from build123d import *

# Parameters (mm, degrees)
BOSS_EXTRUDE1_DEPTH = 10
CUT_EXTRUDE4_DEPTH  = 5
SKETCH7_R           = 4.5
CUT_EXTRUDE5_DEPTH  = 5
CUT_EXTRUDE6_DEPTH  = 10
CUT_EXTRUDE7_START  = -2
CUT_EXTRUDE7_DEPTH  = 2
SKETCH11_R          = 2.5
CUT_EXTRUDE8_DEPTH  = 104.25938214


with BuildPart() as part:
    # Sketch1 → Boss-Extrude1 (new body)
    with BuildSketch(Plane(origin=(0, 0, 0), x_dir=(1, 0, 0), z_dir=(0, 1, 0))):
        with BuildLine():
            Line((-32.5, 65), (-32.5, -65))
            ThreePointArc((-32.5, -65), (0, -97.5), (32.5, -65))
            Line((32.5, -65), (32.5, 65))
            ThreePointArc((32.5, 65), (0, 97.5), (-32.5, 65))
        make_face()
    extrude(amount=BOSS_EXTRUDE1_DEPTH)

    # Sketch6 → Cut-Extrude4 (cut)
    with BuildSketch(Plane(origin=(0, 10, 0), x_dir=(1, 0, 0), z_dir=(0, 1, 0))):
        with BuildLine():
            Line((-25, -65), (-25, 25))
            Line((-25, 25), (25, 25))
            Line((25, 25), (25, -65))
            ThreePointArc((25, -65), (0, -90), (-25, -65))
        make_face()
    extrude(amount=-CUT_EXTRUDE4_DEPTH, mode=Mode.SUBTRACT)

    # Sketch7 → Cut-Extrude5 (cut)
    with BuildSketch(Plane(origin=(0, 5, 0), x_dir=(1, 0, 0), z_dir=(0, 1, 0))):
        with Locations(Location((0, -65, 0), (0, 0, 270))):
            Circle(SKETCH7_R)
    extrude(amount=-CUT_EXTRUDE5_DEPTH, mode=Mode.SUBTRACT)

    # Sketch8 → Cut-Extrude6 (cut)
    with BuildSketch(Plane(origin=(0, 5, 0), x_dir=(1, 0, 0), z_dir=(0, 1, 0))):
        with BuildLine():
            Line((-16, -65), (-11, -65))
            ThreePointArc((-11, -65), (-7.778174593, -72.778174593), (0, -76))
            Line((0, -76), (0, -81))
            ThreePointArc((0, -81), (-11.313708499, -76.313708499), (-16, -65))
        make_face()
    extrude(amount=-CUT_EXTRUDE6_DEPTH, mode=Mode.SUBTRACT)

    # Sketch9 → Cut-Extrude7 (cut)
    with BuildSketch(Plane(origin=(0, 10, 0), x_dir=(1, 0, 0), z_dir=(0, 1, 0)).offset(CUT_EXTRUDE7_START)):
        with BuildLine():
            Line((-32.5, -65), (-30.5, -65))
            ThreePointArc((-30.5, -65), (0, -95.5), (30.5, -65))
            Line((30.5, -65), (32.5, -65))
            ThreePointArc((32.5, -65), (0, -97.5), (-32.5, -65))
        make_face()
        with BuildLine():
            Line((-30.5, 65), (-32.5, 65))
            ThreePointArc((-32.5, 65), (0, 97.5), (32.5, 65))
            Line((32.5, 65), (30.5, 65))
            ThreePointArc((30.5, 65), (0, 95.5), (-30.5, 65))
        make_face()
    extrude(amount=CUT_EXTRUDE7_DEPTH, mode=Mode.SUBTRACT)

    # Sketch11 → Cut-Extrude8 (cut, through all)
    with BuildSketch(Plane(origin=(0, 10, 0), x_dir=(1, 0, 0), z_dir=(0, 1, 0))):
        with Locations(Location((26, 32.5, 0), (0, 0, 270))):
            Circle(SKETCH11_R)
        with Locations(Location((-26, 32.5, 0), (0, 0, 270))):
            Circle(SKETCH11_R)
    extrude(amount=-CUT_EXTRUDE8_DEPTH, mode=Mode.SUBTRACT)


solid = part.part
Check sheet for the modelled part. Datum: model origin and axes. Units: mm. A direction names the side the tool comes from. Round coordinates to 2 decimals unless told otherwise and drop trailing zeros. Loops run counter-clockwise (first coordinate to the right, second up) from the corner with the lowest first, then second, coordinate; pieces in that order, holes last. Notation, with made-up numbers: M 79,22 L 101,22 A21 cw 101,50 Z; hole C 69.25,40.5 d4. An arc over 180 degrees is marked long. One line per question, with ' | ' between items. Start each with the question number.
Item 1: Release check for a two-part mould opening along Z. For faces 1 (the face through (-0.671, 8.986, 95.493)), 2 (the face through (-32.5, 5, -1)), 3 (the face through (-23.52, 5.07, -32.83)), 4 (the face through (-11.189, 2.535, 76.437)) record: released by +Z, released by -Z, zero draft, split by the parting line, or undercut.
Item 2: Scan lines: probe 1 along X at (y, z) = (3.25, -32.5); probe 2 along X at (y, z) = (8.25, 3.5); probe 3 along Y at (x, z) = (14.5, 2.5). Record each from-to range of solid material in increasing order.
Item 3: Section check A-A (z = -32.5). Record the boundary of the cut face in (x, y), and give its area (3 significant figures).
Item 4: Set-up check for faces 5 (the face through (0, 3, 78)), 6 (the face through (0, 8, 96)), 7 (the face through (0.55, 7.535, 89.994)), 8 (the face through (0.671, 8.986, -95.493)): record each of +Z, -Z, +X, -X, +Y, -Y from which the full face is reachable in a straight line by a thin tool's end or side.
Item 5: Section check B-B (x = -13). Record the boundary of the cut face in (y, z), and give its area (3 significant figures).
Item 6: Section check C-C (z = -67.5). Record the boundary of the cut face in (x, y), and give its area (3 significant figures).
Item 7: Gauge pin test, flat ends, axial feed: pin 1 Ø5 at (x, y) = (-13.5, 7.5) entering from +Z; pin 2 Ø4 at (y, z) = (1.5, 78.5) entering from -X; pin 3 Ø5 at (x, y) = (-22, 2) entering from -Z. Record the tip position at first contact, or that the pin passes through.
Worked out:
1) face 1: released by +Z | face 2: zero draft | face 3: undercut | face 4: undercut
2) probe 1: -32.5 to -28.5, -23.5 to 23.5, 28.5 to 32.5 | probe 2: -32.5 to -25, 25 to 32.5 | probe 3: 0 to 5
3) outline: M -32.5,0 L -28.5,0 L -28.5,10 L -32.5,10 Z; M -23.5,0 L 23.5,0 L 23.5,10 L -23.5,10 Z; M 28.5,0 L 32.5,0 L 32.5,10 L 28.5,10 Z | area: 550 mm^2
4) face 5: +Y, -Y | face 6: +Z, +Y | face 7: +Y | face 8: -Z, +Y
5) outline: M 0,-94.79 L 8,-94.79 L 8,-92.59 L 10,-92.59 L 10,-25 L 5,-25 L 5,65 L 0,65 Z; M 0,74.33 L 5,74.33 L 5,86.35 L 10,86.35 L 10,92.59 L 8,92.59 L 8,94.79 L 0,94.79 Z | area: 1,280 mm^2
6) outline: M -32.4,0 L 32.4,0 L 32.4,8 L 30.4,8 L 30.4,10 L -30.4,10 L -30.4,8 L -32.4,8 Z | area: 640 mm^2
7) pin 1: z = 95.58 | pin 2: x = -30.4 | pin 3: z = -91
